Autodesk Inventor part; units mm, degrees
ref_plane "YZ Plane" through (0, 0, 0) normal (1, 0, 0) x (0, 1, 0)
ref_plane "XZ Plane" through (0, 0, 0) normal (0, 1, 0) x (-1, 0, 0)
ref_plane "XY Plane" through (0, 0, 0) normal (0, 0, 1) x (1, 0, 0)
sketch "Sketch1" plane through (0, 0, 0) normal (0, 0, 1) x (1, 0, 0)
  line L0 (-230, 0) -> (230, 0)
  line L1 (230, 0) -> (230, -70)
  line L2 (230, -70) -> (-230, -70)
  line L3 (-230, -70) -> (-230, 0)
  point P0 (0, 0)
  point P1 (0, 0)
  dimension "d0" = 460
  dimension "d1" = 70
extrude "Plate1" add sketch "Sketch1" against normal blind 3
sketch "Sketch2" plane through (0, 0, 0) normal (0, 0, 1) x (1, 0, 0)
  line L0 (-230, -70) -> (230, -70)
  line L1 (230, -70) -> (230, 0)
  line L2 (230, 0) -> (-230, 0)
  line L3 (-230, 0) -> (-230, -70)
  circle A0 centre (0, -63) radius 4
  circle A1 centre (0, -50) radius 4
  line L4 (4, -63) -> (4, -50)
  line L5 (-4, -63) -> (-4, -50)
  point P0 (0, 0)
  point P1 (0, -70)
  dimension "d3" = 8
  dimension "d5" = 7
  dimension "d22" = 13
extrude "Cut1" cut sketch "Sketch2" against normal through all contours A0 | A0 L5 A1 L4 | A1
pattern_linear "Rectangular Pattern1" count 7 spacing 70 along (-1, 0, 0) of "Cut1" first direction both ways yes
sketch "Sketch3" plane through (0, 0, 0) normal (0, 0, 1) x (1, 0, 0)
  line L0 (1.55, -20) -> (-1.55, -20)
  line L1 (-1.55, -20) -> (-1.55, 0)
  line L2 (-1.55, 0) -> (1.55, 0)
  line L3 (1.55, 0) -> (1.55, -20)
  line L4 (230, 0) -> (-230, 0)
  point P0 (0, 0)
  point P1 (0, 0)
  point P2 (0, 0)
  dimension "d11" = 3.1
  dimension "d12" = 20
extrude "Cut2" cut sketch "Sketch3" against normal blind 3
pattern_linear "Rectangular Pattern2" count 3 spacing 173 along (-1, 0, 0) of "Cut2" first direction both ways yes
equation "\"d6\" = Thickness"
equation "\"d13\" = Thickness"
equation "\"d2\" = Thickness"
equation "\"BendReliefWidth\" = Thickness"
equation "\"BendReliefDepth\" = 0.5 * Thickness"
equation "\"CornerReliefSize\" = 4 * Thickness"
equation "\"MinimumRemnant\" = 2 * Thickness"
equation "\"TransitionRadius\" = BendRadius"
equation "\"JacobiRadiusSize\" = BendRadius"
equation "\"GapSize\" = Thickness"
properties part number "TRM 032 plate" material "Stainless Steel"
For this review, take the finished solid that the model builds, in its own axes (mm). Round coordinates to 2 decimals unless told otherwise and drop trailing zeros. Write each loop counter-clockwise with the first axis right and the second up, starting at its lowest first coordinate (ties: lowest second). Pieces come first, ordered by that corner, then holes. Notation, with made-up numbers: M -32.5,-37.5 L -26.5,-37.5 A18 cw -26.5,-33.5 Z; hole C -25.5,69.25 d7. An arc over 180 degrees is marked long. Write item = value, one per line. Start each with the question number.
(1) We need section A-A (x = -70). Give the boundary of the cut face in (y, z), then the cut area to 3 significant figures.
(2) We need section B-B (y = -12). Give the boundary of the cut face in (x, z).
(3) Clearance check with a flat-ended pin moving along its axis: pin 1 Ø0.9 at (x, z) = (172.5, -2) entering from +Y. State where the tip first meets the part, or that it passes through.
(4) For line 1 along X through (y, z) = (-16, -1.3); line 2 along Y through (x, z) = (-137, -0.2), list the stretches that pass through material, from the lowest coordinate up.
(5) We need section C-C (z = -2.2). Give the number of separate pieces and of enclosed holes in the cut face, then the cut area to 3 significant figures.
Results found:
q1.outline = M -70,-3 L -67,-3 L -67,0 L -70,0 Z; M -46,-3 L 0,-3 L 0,0 L -46,0 Z
q1.area = 147 mm²
q2.outline = M -230,-3 L -174.55,-3 L -174.55,0 L -230,0 Z; M -171.45,-3 L -1.55,-3 L -1.55,0 L -171.45,0 Z; M 1.55,-3 L 171.45,-3 L 171.45,0 L 1.55,0 Z; M 174.55,-3 L 230,-3 L 230,0 L 174.55,0 Z
q3.pin_1 = -20
q4.line_1 = -230 to -174.55, -171.45 to -1.55, 1.55 to 171.45, 174.55 to 230
q4.line_2 = -70 to -65.65, -47.35 to 0
q5.separate_pieces = 1
q5.enclosed_holes = 7
q5.area = 30,900 mm²
